Autodesk Fusion 360 part; units mm, degrees
sketch "スケッチ4" plane through (0, 0, 0) normal (1, 0, 0) x (0, 1, 0)
  arc A0 (9.5, 0) -> (-9.5, 0) centre (0, 0) ccw
  line L0 (9.5, 0) -> (9.5, -11.5)
  line L1 (9.5, -11.5) -> (-9.5, -11.5)
  line L2 (-9.5, -11.5) -> (-9.5, 0)
  dimension "d8" = 9.5
  dimension "d9" = 19
  dimension "d10" = 11.5
extrude "押し出し2" add sketch "スケッチ4" along normal mid plane 95
sketch "スケッチ6" plane through (0, 0, 0) normal (1, 0, 0) x (0, 1, 0)
  arc A0 (11, 0) -> (-11, 0) centre (0, 0) ccw
  line L0 (11, 0) -> (11, -9.5)
  line L1 (11, -9.5) -> (-11, -9.5)
  line L2 (-11, -9.5) -> (-11, 0)
  dimension "d17" = 9.5
  dimension "d18" = 22
extrude "押し出し3" add sketch "スケッチ6" along normal mid plane 48
sketch "スケッチ7" plane through (47.5, 0, 0) normal (1, 0, 0) x (0, 1, 0)
  arc A0 (9.5, 0) -> (-9.5, 0) centre (0, 0) ccw
  line L0 (-9.5, 0) -> (-9.5, -11.5)
  line L1 (-9.5, -11.5) -> (9.5, -11.5)
  line L2 (9.5, -11.5) -> (9.5, 0)
  circle A1 centre (0, 0) radius 4.75
  dimension "d21" = 9.5
extrude "押し出し4" cut sketch "スケッチ7" along normal through all and the other way through all contours A1
Verification items for the finished model (mm, model axes). A direction names the side the tool comes from. Give positions to 0.01 mm unless a question says otherwise; leave off trailing zeros. Write each loop counter-clockwise with the first axis right and the second up, starting at its lowest first coordinate (ties: lowest second). Pieces come first, ordered by that corner, then holes. Notation, with made-up numbers: M -34,4 L -23,4 A20 cw -23,19 Z; hole C 46.5,18.25 d4. An arc over 180 degrees is marked long. Put each result on its own line as item: value. Start each with the question number.
1. Section check C-C (z = -3.5). Record the cut outline in (x, y).
2. Section check A-A (y = 0). Record the cut outline in (x, z), and give its area (3 significant figures).
3. Set-up check for faces 5 (the face through (24, -6, 8)), 6 (the face through (47.5, 0, -6)), 7 (the face through (-35.915, -0.209, 9.498)): record each of +Z, -Z, +X, -X, +Y, -Y from which the full face is reachable in a straight line by a thin tool's end or side.
4. Go/stop test with flat-tipped pins: pin 1 Ø4 at (x, z) = (31.5, -7.5) entering from +Y; pin 2 Ø4 at (x, z) = (6.5, 5.5) entering from -Y; pin 3 Ø0.8 at (x, y) = (-10, 10.5) entering from -Z; pin 4 Ø10 at (y, z) = (-4, -1) entering from -X. Record where each tip stops, or that it passes through.
5. Scan lines: line 1 along Z through (x, y) = (-16, 0); line 2 along Y through (x, z) = (-14.5, 2.25); line 3 along Z through (x, y) = (4.5, -1.75). Record each from-to range of solid material in increasing order. Write a range as [from, to].
6. Draft check along Z on faces 1 (the face through (-47.5, 0, -6)), 2 (the face through (-1, 0, -11.5)), 3 (the face through (0.665, 2.192, -4.214)), 4 (the face through (35.585, -0.209, 9.498)). Enter one of: +Z half, -Z half, draft (parallel to the pull), parting line (faces both ways), or undercut.
7. Section check B-B (x = 20). Record the cut outline in (y, z).
8. Section check D-D (x = -29.5). Record the cut outline in (y, z), and give its area (3 significant figures).
Answer list:
1. outline: M -47.5,-9.5 L -24,-9.5 L -24,-11 L 24,-11 L 24,-9.5 L 47.5,-9.5 L 47.5,-3.21 L -47.5,-3.21 Z; M -47.5,3.21 L 47.5,3.21 L 47.5,9.5 L 24,9.5 L 24,11 L -24,11 L -24,9.5 L -47.5,9.5 Z
2. outline: M -47.5,-11.5 L 47.5,-11.5 L 47.5,-4.75 L -47.5,-4.75 Z; M -47.5,4.75 L 47.5,4.75 L 47.5,9.5 L 24,9.5 L 24,11 L -24,11 L -24,9.5 L -47.5,9.5 Z
2. area: 1,160 mm2
3. face 5: +Z, +X
3. face 6: +Z, -Z, +X, +Y, -Y
3. face 7: +Z, -X
4. pin 1: y = 9.5
4. pin 2: y = -10.43
4. pin 3: z = -9.5
4. pin 4: x = -47.5
5. line 1: [-11.5, -4.75], [4.75, 11]
5. line 2: [-10.77, -4.18], [4.18, 10.77]
5. line 3: [-11.5, -4.42], [4.42, 10.86]
6. face 1: draft
6. face 2: -Z half
6. face 3: undercut
6. face 4: +Z half
7. outline: M -11,-9.5 L -9.5,-9.5 L -9.5,-11.5 L 9.5,-11.5 L 9.5,-9.5 L 11,-9.5 L 11,0 A11 ccw -11,0 Z; hole C 0,0 d9.5
8. outline: M -9.5,-11.5 L 9.5,-11.5 L 9.5,0 A9.5 ccw -9.5,0 Z; hole C 0,0 d9.5
8. area: 289 mm2
